Check sheet for the drawn part. Datum: minimum x, y, z corner. Units: mm. A direction names the side the tool comes from. Coordinates: 2 decimals unless noted, no trailing zeros. Write each loop counter-clockwise with the first axis right and the second up, starting at its lowest first coordinate (ties: lowest second). Pieces come first, ordered by that corner, then holes. Notation, with made-up numbers: (48, 1) - (68, 1) arc R20 cw to (68, 23) - close; hole circle Ø10 at (-39, 62.25). An arc over 180 degrees is marked (long way). Use one line per item in the form item = value. Start each with the question number.
1. Go/stop test with flat-tipped pins: pin 1 Ø3 at (x, y) = (21.5, 5) entering from -Z; pin 2 Ø3 at (x, y) = (2.5, 3.5) entering from -Z; pin 3 Ø1.5 at (x, y) = (26.5, 1.5) entering from -Z. Record where each tip stops, or that it passes through.
2. Scan lines: line 1 along X through (y, z) = (2.5, 9.5) (1 decimal); line 2 along Z through (x, y) = (5, 3.3); line 3 along Z through (x, y) = (23.5, 2.05). Record each from-to range of solid material in increasing order.
3. Tool access check on the marked faces 1, 2 and 3. Record the directions out of +Z, -Z, +X, -X, +Y, -Y that give a thin tool (end or side, any length) a straight path to the whole face; none if there is none.
4. Cross-section at B-B on x = 3. Record the boundary of the cut face in (y, z).
5. Cross-section at C-C on z = 14. Record the boundary of the cut face in (x, y), then the cut area to 3 significant figures.
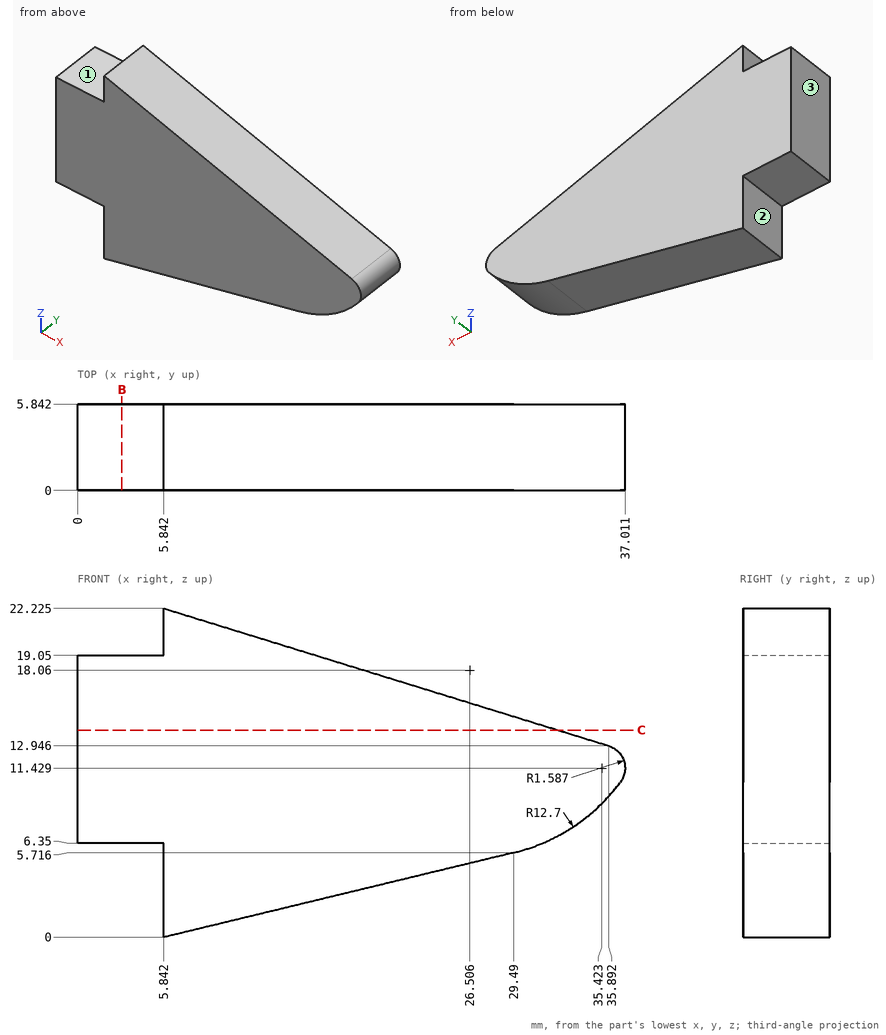
Final values:
q1.pin_1 = 3.42
q1.pin_2 = 6.35
q1.pin_3 = 4.81
q2.line_1 = 0 to 35.9
q2.line_2 = 6.35 to 19.05
q2.line_3 = 4.27 to 16.77
q3.face_1 = +Z, -X, +Y, -Y
q3.face_2 = -Z, -X, +Y, -Y
q3.face_3 = +Z, -Z, -X, +Y, -Y
q4.outline = (0, 6.35) - (5.84, 6.35) - (5.84, 19.05) - (0, 19.05) - close
q5.outline = (0, 0) - (32.48, 0) - (32.48, 5.84) - (0, 5.84) - close
q5.area = 190 mm²
